Design review of the part built by this model. Coordinates are the model's own, in mm. A direction names the side the tool comes from. Coordinates: 2 decimals unless noted, no trailing zeros. Loops run counter-clockwise (first coordinate to the right, second up) from the corner with the lowest first, then second, coordinate; pieces in that order, holes last. Notation, with made-up numbers: (20.25, 9) -> (69.25, 9) arc R25 ccw to (69.25, 29) -> close; hole circle Ø4 at (38, -24.75). An arc over 180 degrees is marked (long way). Answer in a Markdown table with one row per item.
```python
from build123d import *

# Parameters (mm, degrees)
BOSS_EXTRU_1_DEPTH                                = 10
ESQUISSE2_R                                       = 5.000000000000001
ENL_V_MAT_EXTRU_1_DEPTH                           = 59.16945460210114
ENL_V_MAT_EXTRU_5_DEPTH                           = 6
D_GAGEMENT_M3_52_D                                = 3.7
D_GAGEMENT_M3_52_DEPTH                            = 3
D_GAGEMENT_M3_52_TIP                              = 1.1115921452009865
ESQUISSE16_W                                      = 32.38443417416177
ESQUISSE16_H                                      = 29.10998154186418
ENL_V_MAT_EXTRU_6_DEPTH                           = 5
CHAMBRAGE_POUR_VIS_T_TE_HEXAGONALE_M3_D           = 3.2
CHAMBRAGE_POUR_VIS_T_TE_HEXAGONALE_M3_CBORE_D     = 8.412
CHAMBRAGE_POUR_VIS_T_TE_HEXAGONALE_M3_CBORE_DEPTH = 2
SKETCH1_R                                         = 1.8499999999999994
SKETCH1_R_2                                       = 1.8499999999999885
SKETCH1_R_3                                       = 5.5
BOSS_EXTRUDE1_DEPTH                               = 8


with BuildPart() as part:
    # Esquisse1 → Boss.-Extru.1 (new body)
    with BuildSketch(Plane.XY):
        with BuildLine():
            Line((-30.751266961285342, 21.842240344710792), (1.248733038714648, 21.842240344710792))
            Line((1.248733038714648, 21.842240344710792), (29.248733038714647, 21.842240344710792))
            Line((29.248733038714647, 21.842240344710792), (29.24873303871465, 3.8422403447107913))
            ThreePointArc((29.24873303871465, 3.8422403447107913), (41.24873303871465, -8.157759655289208), (29.24873303871465, -20.157759655289208))
            Line((29.24873303871465, -20.157759655289208), (29.248733038714654, -38.15775965528921))
            Line((29.248733038714654, -38.15775965528921), (-30.751266961285342, -38.15775965528921))
            Line((-30.751266961285342, -38.15775965528921), (-30.751266961285346, -20.157759655289208))
            ThreePointArc((-30.751266961285346, -20.157759655289208), (-42.75126696128535, -8.15775965528921), (-30.751266961285346, 3.8422403447107913))
            Line((-30.751266961285346, 3.8422403447107913), (-30.751266961285342, 21.842240344710792))
        make_face()
    extrude(amount=BOSS_EXTRU_1_DEPTH)

    # Esquisse2 → Enlèv. mat.-Extru.1 (cut, through all)
    with BuildSketch(Plane.XY.offset(10)):
        with Locations((-0.7512669612853434, -8.157759655289208)):
            Circle(ESQUISSE2_R)
    extrude(amount=-ENL_V_MAT_EXTRU_1_DEPTH, mode=Mode.SUBTRACT)

    # Esquisse13 → Enlèv. mat.-Extru.5 (cut)
    with BuildSketch(Plane(origin=(0, 0, 0), x_dir=(-1, 0, 0), z_dir=(0, 0, -1))):
        Polygon((-27.248733038714654, 19.842240344710792), (28.751266961285335, 19.842240344710792), (28.751266961285346, -36.15775965528921), (-27.248733038714647, -36.15775965528921), align=None)
    extrude(amount=-ENL_V_MAT_EXTRU_5_DEPTH, mode=Mode.SUBTRACT)

    # Dégagement M3.52
    with Locations(Plane(origin=(0, 0, 6), x_dir=(-1, 0, 0), z_dir=(0, 0, -1))):
        with Locations((8.251266961, -8.157759655), (-6.748733039, -8.157759655)):
            Hole(D_GAGEMENT_M3_52_D / 2, depth=D_GAGEMENT_M3_52_DEPTH)
            with Locations((0, 0, -(D_GAGEMENT_M3_52_DEPTH + D_GAGEMENT_M3_52_TIP / 2))):  # 118° drill point
                Cone(0, D_GAGEMENT_M3_52_D / 2, D_GAGEMENT_M3_52_TIP, mode=Mode.SUBTRACT)

    # Esquisse16 → Enlèv. mat.-Extru.6 (cut)
    with BuildSketch(Plane.XY.offset(10)):
        Polygon((-30.75126696128535, 3.8422403447107913), (-47.0482075621835, 3.8422403447107896), (-47.0482075621835, -23.80458867239539), (-30.75126696128535, -23.804588672395386), align=None)
        with Locations((45.44095012579554, -10.712750426221298)):
            Rectangle(ESQUISSE16_W, ESQUISSE16_H)
    extrude(amount=-ENL_V_MAT_EXTRU_6_DEPTH, mode=Mode.SUBTRACT)

    # Chambrage pour vis à tête hexagonale M3 (Grade A)1 (through all)
    with Locations(Plane.XY.offset(5)):
        with Locations((34.748733039, -8.157759655), (-36.251266961, -8.157759655)):
            CounterBoreHole(CHAMBRAGE_POUR_VIS_T_TE_HEXAGONALE_M3_D / 2, CHAMBRAGE_POUR_VIS_T_TE_HEXAGONALE_M3_CBORE_D / 2, CHAMBRAGE_POUR_VIS_T_TE_HEXAGONALE_M3_CBORE_DEPTH)

    # Sketch1 → Boss-Extrude1 (add)
    with BuildSketch(Plane(origin=(0, 0, 6), x_dir=(-1, 0, 0), z_dir=(0, 0, -1))):
        Polygon((-13.248733038714654, -0.15775965528920868), (-13.248733038714652, -16.157759655289208), (14.751266961285353, -16.157759655289208), (14.751266961285348, -0.15775965528920868), align=None)
        with Locations((-6.748733038714656, -8.15775965528921)):
            Circle(SKETCH1_R, mode=Mode.SUBTRACT)
        with Locations((8.251266961285344, -8.15775965528921)):
            Circle(SKETCH1_R_2, mode=Mode.SUBTRACT)
        with Locations((0.7512669612853434, -8.157759655289208)):
            Circle(SKETCH1_R_3, mode=Mode.SUBTRACT)
    extrude(amount=BOSS_EXTRUDE1_DEPTH)


solid = part.part
```
(1) Tool access review of faces 1 (the cylindrical face through (38.634, -9.769, 4.014)), 2 (the flat face through (-1, 21.842, 5)), 3 (the flat face through (31, -5, 5)), 4 (the flat face through (-1, -36.158, 3)): name each direction out of +Z, -Z, +X, -X, +Y, -Y from which nothing blocks a thin tool from reaching the whole face with its end or side.
Evaluation:
| item | result |
|---|---|
| face 1 | +Z |
| face 2 | +Z, -Z, +X, -X, +Y |
| face 3 | +Z, +X, +Y, -Y |
| face 4 | -Z |
(2) To check wall thickness, follow probe 1 along X at (y, z) = (-8, 5.25); probe 2 along Y at (x, z) = (1.5, 3.25); probe 3 along Y at (x, z) = (-0.5, 9). State the ranges of each line that lie inside material, in increasing order.
Evaluation:
| item | result |
|---|---|
| probe 1 | x = -30.75 to -28.75, -14.75 to -10.09, -6.41 to -6.25, 4.75 to 4.91, 8.59 to 13.25, 27.25 to 29.25 |
| probe 2 | y = -38.16 to -36.16, -16.16 to -13.18, -3.14 to -0.16, 19.84 to 21.84 |
| probe 3 | y = -38.16 to -13.15, -3.16 to 21.84 |
(3) Take a section at B-B on z = 4. Give the boundary of the cut face in (x, y).
Evaluation:
| item | result |
|---|---|
| outline | (-30.75, -38.16) -> (29.25, -38.16) -> (29.25, -20.16) arc R12 ccw to (29.25, 3.84) -> (29.25, 21.84) -> (-30.75, 21.84) -> (-30.75, 3.84) arc R12 ccw to (-30.75, -20.16) -> close; (-14.75, -16.16) -> (13.25, -16.16) -> (13.25, -0.16) -> (-14.75, -0.16) -> close; hole circle Ø8.41 at (-36.25, -8.16); hole (-28.75, -36.16) -> (27.25, -36.16) -> (27.25, 19.84) -> (-28.75, 19.84) -> close; hole circle Ø3.7 at (-8.25, -8.16); hole circle Ø11 at (-0.75, -8.16); hole circle Ø3.7 at (6.75, -8.16); hole circle Ø8.41 at (34.75, -8.16) |
(4) Draft analysis for pull direction X (two halves, no side actions). For faces 5 (the cylindrical face through (-34.653, -8.087, 1.479)), 6 (the flat face through (27.4, -8, 0)), state which applies: pulls with the +X half, pulls with the -X half, needs draft (parallel to the pull), parting line crosses it, or undercut.
Evaluation:
| item | result |
|---|---|
| face 5 | undercut |
| face 6 | needs draft |
(5) Take a section at C-C on y = -26. Give the boundary of the cut face in (x, z), and give its area (3 significant figures).
Evaluation:
| item | result |
|---|---|
| outline | (-30.75, 0) -> (-28.75, 0) -> (-28.75, 6) -> (27.25, 6) -> (27.25, 0) -> (29.25, 0) -> (29.25, 10) -> (-30.75, 10) -> close |
| area | 264 mm² |
(6) Take a section at D-D on x = -17. Give the boundary of the cut face in (y, z).
Evaluation:
| item | result |
|---|---|
| outline | (-38.16, 0) -> (-36.16, 0) -> (-36.16, 6) -> (19.84, 6) -> (19.84, 0) -> (21.84, 0) -> (21.84, 10) -> (-38.16, 10) -> close |
(7) Take a section at A-A on x = 1. Give the boundary of the cut face in (y, z).
Evaluation:
| item | result |
|---|---|
| outline | (-38.16, 0) -> (-36.16, 0) -> (-36.16, 6) -> (-16.16, 6) -> (-16.16, -2) -> (-13.37, -2) -> (-13.37, 6) -> (-12.84, 6) -> (-12.84, 10) -> (-38.16, 10) -> close; (-3.47, 6) -> (-2.94, 6) -> (-2.94, -2) -> (-0.16, -2) -> (-0.16, 6) -> (19.84, 6) -> (19.84, 0) -> (21.84, 0) -> (21.84, 10) -> (-3.47, 10) -> close |
(8) For pin 1 (5 mm diameter, centred on x = 34.75, y = -8.16, fed in from +Z); pin 2 (8 mm diameter, centred on x = -5, y = -27.5, fed in from -Z); pin 3 (1.5 mm diameter, centred on y = -13.5, z = 1.5, fed in from +X), all flat-tipped, find the tip position at first contact; note any pin that passes through.
Evaluation:
| item | result |
|---|---|
| pin 1 | stops at z = 3 |
| pin 2 | stops at z = 6 |
| pin 3 | stops at x = 40.34 |
